from build123d import *

# Parameters (mm, degrees)
F2_SIZE  = 2.54
F3_SIZE  = 1.27
F5_DEPTH = 1.27
F6_R     = 1.5
F7_DEPTH = 10
F8_W     = 32.420068
F8_H     = 3.81
F9_DEPTH = 3.81


with BuildPart() as f1:
    # F0 (on Front) → F1 (revolve)
    with BuildSketch(Plane.XZ):
        Polygon((-40.64, 0), (-57.15, 0), (-57.15, -20.574), (-46.101, -20.574), (-46.101, -25.654), (-3.5, -25.654), (-3.5, -22.225), (-40.64, -22.225), align=None)
    revolve(axis=Axis((0, 0, 19.796192), (0, 0, -1)))

    # F2
    f2_edges = [f1.edges().sort_by_distance(p)[0] for p in [
        (57.15, 0, -20.574),
    ]]
    chamfer(f2_edges, length=F2_SIZE)

    # F3
    f3_edges = [f1.edges().sort_by_distance(p)[0] for p in [
        (46.101, 0, -25.654),
    ]]
    chamfer(f3_edges, length=F3_SIZE)

    # F4 (on face) → F5 (cut)
    with BuildSketch(Plane.XY.offset(-22.225)):
        with BuildLine():
            Line((5.2324, 6.731), (-5.2324, 6.731))
            ThreePointArc((-5.2324, 6.731), (-7.183623, 7.539223), (-6.3754, 5.588))
            Line((-6.3754, 5.588), (-6.3754, -5.588))
            ThreePointArc((-6.3754, -5.588), (-7.183623, -7.539223), (-5.2324, -6.731))
            Line((-5.2324, -6.731), (5.2324, -6.731))
            ThreePointArc((5.2324, -6.731), (7.183623, -7.539223), (6.3754, -5.588))
            Line((6.3754, -5.588), (6.3754, 5.588))
            ThreePointArc((6.3754, 5.588), (7.183623, 7.539223), (5.2324, 6.731))
        make_face()
    extrude(amount=-F5_DEPTH, mode=Mode.SUBTRACT)

    # F6 (on face) → F7 (cut)
    with BuildSketch(Plane.XY):
        with Locations((-48.895, 0)):
            Circle(F6_R)
        with Locations((24.4475, -42.344312)):
            Circle(F6_R)
        with Locations((24.4475, 42.344312)):
            Circle(F6_R)
    extrude(amount=-F7_DEPTH, mode=Mode.SUBTRACT)

    # F8 (on face) → F9 (cut)
    with BuildSketch(Plane.XY):
        with Locations((49.065037, 0)):
            Rectangle(F8_W, F8_H)
    extrude(amount=-F9_DEPTH, mode=Mode.SUBTRACT)


solid = f1.part
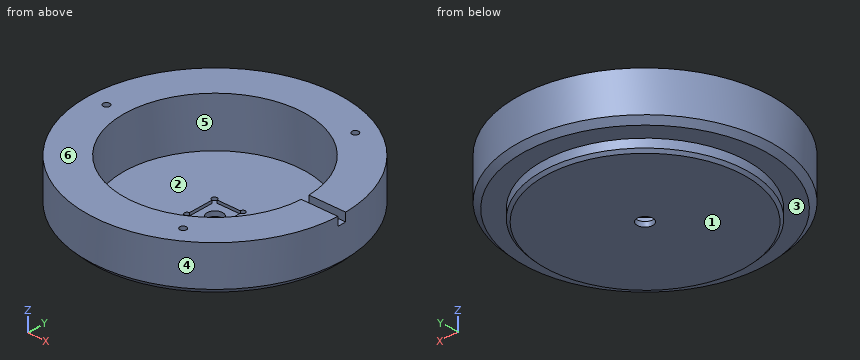
Source: CAD feature listing. Evaluate the final solid. Frame: model axes, mm. Face numbers are marked on the shaded views. A direction names the side the tool comes from. Round coordinates to 2 decimals unless told otherwise and drop trailing zeros. Loops run counter-clockwise (first coordinate to the right, second up) from the corner with the lowest first, then second, coordinate; pieces in that order, holes last. Notation, with made-up numbers: (30.5, 48) - (69.5, 48) arc R30 cw to (69.5, 73) - close; hole circle Ø10 at (57.5, -23). An arc over 180 degrees is marked (long way). Write item = value, one per line. Start each with the question number.
Item 1: Material intervals for line 1 (Y direction, x = 0, z = -5); line 2 (Y direction, x = 24.5, z = -5.5); line 3 (Y direction, x = 0, z = -24.05), sorted ascending.
Item 2: First-contact query: pin 1 Ø10 at (y, z) = (29, -12.5) entering from +X; pin 2 Ø3 at (x, z) = (52, -1.5) entering from +Y; pin 3 Ø2.5 at (x, y) = (24.45, 42.34) entering from +Z. Flat tips, straight axial feed; report the tip coordinate or a pass-through.
Item 3: Mould query, pull axis Y, two halves, no side actions, for the marked faces 4, 5 and 6. Classes: released by +Y, released by -Y, zero draft, split by the parting line, or undercut.
Item 4: Reachability of the marked faces 1, 2 and 3 from +Z, -Z, +X, -X, +Y, -Y: full face, straight path, thin tool, end or side. Return the list, or none.
Item 5: Section query B-B on x = 0. Output: boundary loops of the cut face in (y, z) (3 decimals), plus the area to 3 significant figures.
Item 6: Section query C-C on z = -8.25. Count the separate pieces of the cut face and the enclosed holes in it, plus the area to 3 significant figures.
Item 7: Section query A-A on y = 0. Output: boundary loops of the cut face in (x, z) (3 decimals), plus the area to 3 significant figures.
Results list:
q1.line_1 = -57.15 to -40.64, 40.64 to 57.15
q1.line_2 = -51.63 to -43.84, -40.85 to -32.42, 32.42 to 40.85, 43.84 to 51.63
q1.line_3 = -46.1 to -3.5, 3.5 to 46.1
q2.pin_1 = 51.87
q2.pin_2 = 26.76
q2.pin_3 = -10
q3.face_4 = split by the parting line
q3.face_5 = undercut
q3.face_6 = zero draft
q4.face_1 = -Z, +X, -X, +Y, -Y
q4.face_2 = +Z
q4.face_3 = -Z
q5.outline = (-57.15, -18.034) - (-54.61, -20.574) - (-46.101, -20.574) - (-46.101, -24.384) - (-44.831, -25.654) - (-3.5, -25.654) - (-3.5, -23.495) - (-6.731, -23.495) - (-6.731, -22.225) - (-40.64, -22.225) - (-40.64, 0) - (-57.15, 0) - close; (3.5, -25.654) - (44.831, -25.654) - (46.101, -24.384) - (46.101, -20.574) - (54.61, -20.574) - (57.15, -18.034) - (57.15, 0) - (40.64, 0) - (40.64, -22.225) - (6.731, -22.225) - (6.731, -23.495) - (3.5, -23.495) - close
q5.area = 973 mm²
q6.separate_pieces = 1
q6.enclosed_holes = 4
q6.area = 5,050 mm²
q7.outline = (-57.15, -18.034) - (-54.61, -20.574) - (-46.101, -20.574) - (-46.101, -24.384) - (-44.831, -25.654) - (-3.5, -25.654) - (-3.5, -23.495) - (-6.375, -23.495) - (-6.375, -22.225) - (-40.64, -22.225) - (-40.64, 0) - (-47.395, 0) - (-47.395, -10) - (-50.395, -10) - (-50.395, 0) - (-57.15, 0) - close; (3.5, -25.654) - (44.831, -25.654) - (46.101, -24.384) - (46.101, -20.574) - (54.61, -20.574) - (57.15, -18.034) - (57.15, -3.81) - (40.64, -3.81) - (40.64, -22.225) - (6.375, -22.225) - (6.375, -23.495) - (3.5, -23.495) - close
q7.area = 881 mm²
